```python
from build123d import *

# Parameters (mm, degrees)
BOSS_EXTRUDE2_DEPTH      = 7.35
BOSS_EXTRUDE2_DEPTH_BACK = 7.35
SKETCH2_W                = 15.7
SKETCH2_H                = 15.7
SKETCH3_R                = 8
BOSS_EXTRUDE3_DEPTH      = 20.55
SKETCH4_R                = 7.55
BOSS_EXTRUDE4_DEPTH      = 25.9
BOSS_EXTRUDE5_DEPTH      = 10


with BuildPart() as part:
    # Sketch2 → Boss-Extrude2 (new, two sides: drawn at the far end of the back side and taken through both)
    with BuildSketch(Plane(origin=(0, 0, 0), x_dir=(1, 0, 0), z_dir=(0, 1, 0)).offset(-BOSS_EXTRUDE2_DEPTH_BACK)):
        Rectangle(SKETCH2_W, SKETCH2_H)
    extrude(amount=BOSS_EXTRUDE2_DEPTH + BOSS_EXTRUDE2_DEPTH_BACK)

    # Sketch3 → Boss-Extrude3 (add)
    with BuildSketch(Plane(origin=(7.85, 0, 0), x_dir=(0, 0, -1), z_dir=(1, 0, 0))):
        with Locations(Location((-0.75, 0, 0), (0, 0, 152.560759849))):
            Circle(SKETCH3_R)
    boss_extrude3 = extrude(amount=BOSS_EXTRUDE3_DEPTH)

    # Sketch4 → Boss-Extrude4 (add)
    with BuildSketch(Plane(origin=(0, 0, -7.85), x_dir=(-1, 0, 0), z_dir=(0, 0, -1))):
        with Locations(Location((0, 0, 0), (0, 0, 103.217293988))):
            Circle(SKETCH4_R)
    extrude(amount=BOSS_EXTRUDE4_DEPTH)

    # Sketch5 → Boss-Extrude5 (add)
    with BuildSketch(Plane(origin=(0, 0, -33.75), x_dir=(-1, 0, 0), z_dir=(0, 0, -1))):
        Polygon((-15.532193585, 0), (-10.572107213, -10.198544939), (25.717504309, -7.313596743), (28.4, 0), (25.717504309, 7.313596743), (-10.572107213, 10.198544939), align=None)
    extrude(amount=-BOSS_EXTRUDE5_DEPTH)

    # Mirror1: Boss-Extrude3 across plane
    add(boss_extrude3.mirror(Plane(origin=(0, 0, 0), x_dir=(0, 0, 1), z_dir=(1, 0, 0))))


solid = part.part
```
Geometry check sheet. Reference: the model listing, model coordinates, mm. A direction names the side the tool comes from. Round coordinates to 2 decimals unless told otherwise and drop trailing zeros. Write each loop counter-clockwise with the first axis right and the second up, starting at its lowest first coordinate (ties: lowest second). Pieces come first, ordered by that corner, then holes. Notation, with made-up numbers: (85.5, 65.5) - (103.5, 65.5) arc R21 ccw to (103.5, 92.5) - close; hole circle Ø4 at (64, -33). An arc over 180 degrees is marked (long way). Write each question's results on one line, items separated by ' | '.
(1) Sectioned sample at B-B, the plane x = -16. Enter the section's corners in (y, z).
Computed:
outline: (-8.09, -33.75) - (8.09, -33.75) - (8.09, -23.75) - (-8.09, -23.75) - close; circle Ø16 at (0, 0.75)
(2) Sectioned sample at C-C, the plane y = -6. Enter the section's corners in (x, z).
Computed:
outline: (-28.4, -4.54) - (-7.85, -4.54) - (-7.85, -7.85) - (-4.58, -7.85) - (-4.58, -23.75) - (-26.2, -23.75) - (-26.2, -33.75) - (12.61, -33.75) - (12.61, -23.75) - (4.58, -23.75) - (4.58, -7.85) - (7.85, -7.85) - (7.85, -4.54) - (28.4, -4.54) - (28.4, 6.04) - (7.85, 6.04) - (7.85, 7.85) - (-7.85, 7.85) - (-7.85, 6.04) - (-28.4, 6.04) - close
(3) Set-up check for faces 4 (the face through (13.017, 5.171, -28.82)), 5 (the face through (0, 0, 7.85)), 6 (the face through (7.85, 6, 7)), 7 (the face through (-7.319, -8.776, -28.82)): record each of +Z, -Z, +X, -X, +Y, -Y from which the full face is reachable in a straight line by a thin tool's end or side.
Computed:
face 4: -Z, +X, +Y | face 5: +Z, +Y, -Y | face 6: +Z, +X, +Y | face 7: -Z, -X, -Y
(4) Draft check along Z on faces 1 (the face through (-6, 0, -33.75)), 2 (the face through (17.98, 1.38, 8.63)), 3 (the face through (-7.85, -6, 7)). Enter one of: pulls with the +Z half, pulls with the -Z half, needs draft (parallel to the pull), parting line crosses it, or undercut.
Computed:
face 1: pulls with the -Z half | face 2: undercut | face 3: needs draft
(5) Sectioned sample at A-A, the plane z = -26.5. Enter the section's corners in (x, y).
Computed:
outline: (-28.4, 0) - (-25.72, -7.31) - (10.57, -10.2) - (15.53, 0) - (10.57, 10.2) - (-25.72, 7.31) - close
(6) Sectioned sample at D-D, the plane z = 0.75. Enter the section's corners in (x, y), plus the area to 3 significant figures.
Computed:
outline: (-28.4, -8) - (-7.85, -8) - (-7.85, -7.35) - (7.85, -7.35) - (7.85, -8) - (28.4, -8) - (28.4, 8) - (7.85, 8) - (7.85, 7.35) - (-7.85, 7.35) - (-7.85, 8) - (-28.4, 8) - close | area: 888 mm^2
(7) Depth check by flat-ended pin: pin 1 Ø1.5 at (x, y) = (5.5, -6.5) entering from +Z; pin 2 Ø1.5 at (y, z) = (4.5, -27.5) entering from +X; pin 3 Ø4 at (x, z) = (4, -17.5) entering from +Y. Enter the tip coordinate at first touch or a pass-through.
Computed:
pin 1: stops at z = 7.85 | pin 2: stops at x = 13.71 | pin 3: stops at y = 7.28
(8) Thickness scan on probe 1 along Z at (x, y) = (-21.5, -0.25); probe 2 along Y at (x, z) = (3.5, -5); probe 3 along Z at (x, y) = (-20, 2.25). Record the ranges inside material, lowest first. Write a range as from..to.
Computed:
probe 1: z = -33.75..-23.75, -7.25..8.75 | probe 2: y = -7.35..7.35 | probe 3: z = -33.75..-23.75, -6.93..8.43
